Part model, mm, in its own coordinate system. Face numbers are marked on the shaded views. A direction names the side the tool comes from. Round coordinates to 2 decimals unless told otherwise and drop trailing zeros. Write each loop counter-clockwise with the first axis right and the second up, starting at its lowest first coordinate (ties: lowest second). Pieces come first, ordered by that corner, then holes.
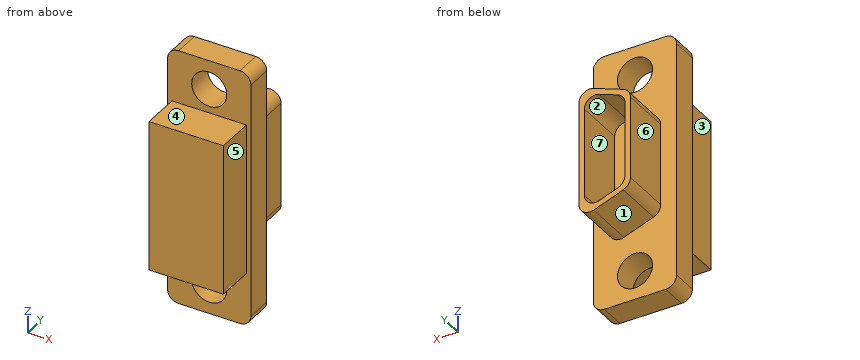
Autodesk Inventor part; units mm, degrees
ref_plane "YZ Plane" through (0, 0, 0) normal (1, 0, 0) x (0, 1, 0)
ref_plane "XZ Plane" through (0, 0, 0) normal (0, 1, 0) x (-1, 0, 0)
ref_plane "XY Plane" through (0, 0, 0) normal (0, 0, 1) x (1, 0, 0)
sketch "Sketch1" plane through (0, 0, 0) normal (0, 1, 0) x (-1, 0, 0)
  line L0 (3.8, 11.75) -> (-3.8, 11.75)
  line L1 (-3.8, 11.75) -> (-3.8, -11.75)
  line L2 (-3.8, -11.75) -> (3.8, -11.75)
  line L3 (3.8, -11.75) -> (3.8, 11.75)
  circle A0 centre (0, 9.1) radius 1.6
  circle A1 centre (0, -9.1) radius 1.6
  point P0 (0, 0)
  dimension "d0" = 23.5
  dimension "d1" = 7.6
  dimension "d2" = 11.75
  dimension "d3" = 3.8
  dimension "d4" = 3.2
  dimension "d5" = 3.2
  dimension "d6" = 18.2
  dimension "d7" = 9.1
extrude "Extrusion1" add sketch "Sketch1" along normal blind 2.4
fillet "Fillet1" radius 1 4 edges at (3.8, 1.2, 11.75) (-3.8, 1.2, 11.75) (3.8, 1.2, -11.75) (-3.8, 1.2, -11.75)
sketch "Sketch2" plane through (0, 2.4, 0) normal (0, 1, 0) x (1, 0, 0)
  line L0 (-2.35, -4.4313) -> (-2.35, 4.4313)
  line L1 (-2.35, 4.4313) -> (2.35, 6.15)
  line L2 (2.35, 6.15) -> (2.35, -6.15)
  line L3 (2.35, -6.15) -> (-2.35, -4.4313)
  line L4 (1.85, -5.4348) -> (-1.85, -4.0818)
  line L5 (-1.85, -4.0818) -> (-1.85, 4.0818)
  line L6 (-1.85, 4.0818) -> (1.85, 5.4348)
  line L7 (1.85, 5.4348) -> (1.85, -5.4348)
  point P0 (0, 0)
  dimension "d11" = 69.914
  dimension "d13" = 12.3
  dimension "d14" = 4.7
  dimension "d15" = 2.35
  dimension "d17" = 0.5
  dimension "d18" = 0.5
  dimension "d19" = 0.5
  dimension "d20" = 0.5
  dimension "d21" = 6.15
  dimension "d22" = 69.914
  dimension "d23" = 69.914
extrude "Extrusion2" add sketch "Sketch2" along normal blind 4.6
fillet "Fillet2" radius 1 8 edges at (-2.35, 4.7, -4.4313) (-2.35, 4.7, 4.4313) (2.35, 4.7, 6.15) (2.35, 4.7, -6.15) (-1.85, 4.7, -4.0818) (-1.85, 4.7, 4.0818) (1.85, 4.7, -5.4348) (1.85, 4.7, 5.4348)
sketch "Sketch3" plane through (0, 0, 0) normal (0, -1, 0) x (1, 0, 0)
  line L0 (3.4, 6.9) -> (-3.4, 6.9)
  line L1 (-3.4, 6.9) -> (-3.4, -6.9)
  line L2 (-3.4, -6.9) -> (3.4, -6.9)
  line L3 (3.4, -6.9) -> (3.4, 6.9)
  point P0 (0, 0)
  dimension "d27" = 13.8
  dimension "d28" = 6.8
  dimension "d29" = 6.9
  dimension "d30" = 3.4
extrude "Extrusion3" add sketch "Sketch3" along normal blind 3.5
equation "\"d5\" = d4"
equation "\"d22\" = d11"
properties part number "15pin male connector"
Q1. Saw through at D-D, the plane z = -9.1. Write the cut outline in (x, y).
Q2. Saw through at B-B, the plane z = -2. Write the cut outline in (x, y), and give its area (3 significant figures).
Q3. Drop flat-ended pins along their axis: P1, Ø3, axis at x = 0.5, y = -2.5, coming from the +Z side; P2, Ø3, axis at y = 4, z = -1, coming from the -X side; P3, Ø3, axis at x = 0, z = -9.1, coming from the -Y side; P4, Ø3.5, axis at y = 5, z = 0.5, coming from the +X side. Give the stop position or say it passes through.
Q4. Tool access for the marked faces 1, 2, 3 and 4: list every direction of +Z, -Z, +X, -X, +Y, -Y with a clear straight run to the whole face (end or side of a thin tool).
Q5. Two-plate mould, pull along X, no slides. Class the marked faces 5, 6 and 7: released by +X, released by -X, zero draft, split by the parting line, or undercut.
Q6. Wall check: line 1 (Z direction, x = 0, y = 0.9); line 2 (Z direction, x = 1, y = 1.5); line 3 (Z direction, x = 0.5, y = -2). Give the ranges that are in metal, low to high.
Q7. Saw through at C-C, the plane x = 0. Write the cut outline in (y, z).
Q8. Saw through at A-A, the plane y = 1. Write the cut outline in (x, z).
Computed:
1. outline: (-3.8, 0) - (-1.6, 0) - (-1.6, 2.4) - (-3.8, 2.4) - close; (1.6, 0) - (3.8, 0) - (3.8, 2.4) - (1.6, 2.4) - close
2. outline: (-3.8, 0) - (-3.4, 0) - (-3.4, -3.5) - (3.4, -3.5) - (3.4, 0) - (3.8, 0) - (3.8, 2.4) - (2.35, 2.4) - (2.35, 7) - (1.85, 7) - (1.85, 2.4) - (-1.85, 2.4) - (-1.85, 7) - (-2.35, 7) - (-2.35, 2.4) - (-3.8, 2.4) - close
2. area: 46.6 mm2
3. P1: stops at z = 6.9
3. P2: stops at x = -2.35
3. P3: passes through
3. P4: stops at x = 2.35
4. face 1: -Z, -X, +Y
4. face 2: +Y
4. face 3: +Z, -Z, -X, -Y
4. face 4: +Z, +X, -X, -Y
5. face 5: released by +X
5. face 6: released by -X
5. face 7: undercut
6. line 1: z = -11.75 to -10.7, -7.5 to 7.5, 10.7 to 11.75
6. line 2: z = -11.75 to -10.35, -7.85 to 7.85, 10.35 to 11.75
6. line 3: z = -6.9 to 6.9
7. outline: (-3.5, -6.9) - (0, -6.9) - (0, -7.5) - (2.4, -7.5) - (2.4, -5.29) - (7, -5.29) - (7, -4.76) - (2.4, -4.76) - (2.4, 4.76) - (7, 4.76) - (7, 5.29) - (2.4, 5.29) - (2.4, 7.5) - (0, 7.5) - (0, 6.9) - (-3.5, 6.9) - close; (0, -11.75) - (2.4, -11.75) - (2.4, -10.7) - (0, -10.7) - close; (0, 10.7) - (2.4, 10.7) - (2.4, 11.75) - (0, 11.75) - close
8. outline: (-3.8, -10.75) arc R1 ccw to (-2.8, -11.75) - (2.8, -11.75) arc R1 ccw to (3.8, -10.75) - (3.8, 10.75) arc R1 ccw to (2.8, 11.75) - (-2.8, 11.75) arc R1 ccw to (-3.8, 10.75) - close; hole circle Ø3.2 at (0, -9.1); hole circle Ø3.2 at (0, 9.1)
